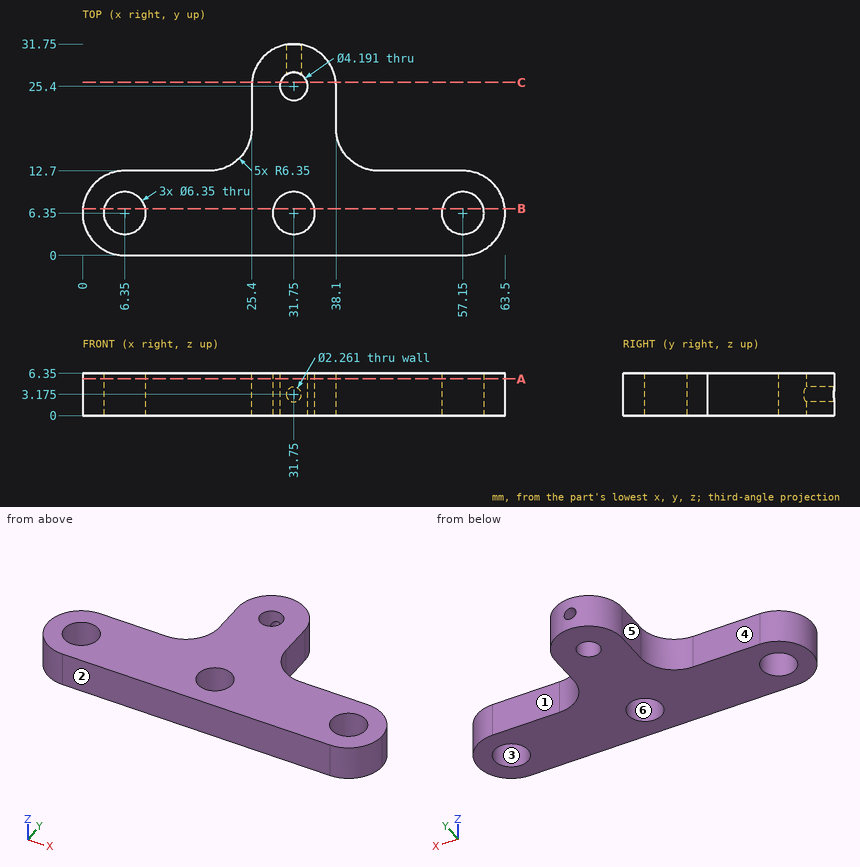
Geometry check sheet. Reference: drawing and pictorial views, mm from the part's lowest x, y, z. A direction names the side the tool comes from. Give positions to 0.01 mm unless a question says otherwise; leave off trailing zeros. Loops run counter-clockwise (first coordinate to the right, second up) from the corner with the lowest first, then second, coordinate; pieces in that order, holes last. Notation, with made-up numbers: (-14.75, 23.25) - (14.25, 23.25) arc R12 ccw to (14.25, 29.25) - close; hole circle Ø10 at (59, 13.5). An arc over 180 degrees is marked (long way). One line per question, with ' | ' between items. Start each with the question number.
1. Set-up check for the marked faces 1 and 2: record each of +Z, -Z, +X, -X, +Y, -Y from which the full face is reachable in a straight line by a thin tool's end or side.
2. Cross-section at B-B, the plane y = 7. Enter the section's corners in (x, z).
3. Gauge pin test, flat ends, axial feed: pin 1 Ø2 at (y, z) = (10.5, 1.5) entering from -X; pin 2 Ø5 at (x, y) = (57.15, 6.35) entering from -Z; pin 3 Ø2 at (x, z) = (56.5, 5) entering from +Y; pin 4 Ø1.5 at (y, z) = (18.5, 1) entering from -X (1 decimal). Record the tip position at first contact, or that the pin passes through.
4. Draft check along X on the marked faces 3, 4, 5 and 6. Enter one of: released by +X, released by -X, zero draft, split by the parting line, or undercut.
5. Cross-section at C-C, the plane y = 26. Enter the section's corners in (x, z).
6. Cross-section at A-A, the plane z = 5.5. Give the number of separate pieces and of enclosed holes in the cut face, plus the area to 3 significant figures.
7. Material ranges on line 1 along X through (y, z) = (7.5, 5.5) (1 decimal); line 2 along Y through (x, z) = (33, 2) (1 decimal); line 3 along Y through (x, z) = (31.75, 3.25) (1 decimal), recorded low to high. Write a range as [from, to].
Check result:
1) face 1: +Z, -Z, +X, +Y | face 2: +Z, -Z, +X, -X, -Y
2) outline: (0.03, 0) - (3.24, 0) - (3.24, 6.35) - (0.03, 6.35) - close; (9.46, 0) - (28.64, 0) - (28.64, 6.35) - (9.46, 6.35) - close; (34.86, 0) - (54.04, 0) - (54.04, 6.35) - (34.86, 6.35) - close; (60.26, 0) - (63.47, 0) - (63.47, 6.35) - (60.26, 6.35) - close
3) pin 1: stops at x = 0.84 | pin 2: passes through | pin 3: stops at y = 12.7 | pin 4: stops at x = 25.3
4) face 3: undercut | face 4: zero draft | face 5: released by -X | face 6: undercut
5) outline: (25.43, 0) - (29.74, 0) - (29.74, 6.35) - (25.43, 6.35) - close; (33.76, 0) - (38.07, 0) - (38.07, 6.35) - (33.76, 6.35) - close
6) separate pieces: 1 | enclosed holes: 4 | area: 905 mm2
7) line 1: x = [0.1, 3.4], [9.3, 28.8], [34.7, 54.2], [60.1, 63.4] | line 2: y = [0, 3.4], [9.3, 23.7], [27.1, 31.6] | line 3: y = [0, 3.2], [9.5, 23.3]
